Drawing for the job (mm, zero at the part's lowest x, y, z). Coordinates: 2 decimals unless noted, no trailing zeros. Order: outer loops, then holes, each group sorted by start corner. A loop starts at its lowest first (then second) coordinate and runs counter-clockwise, first axis right, second up.
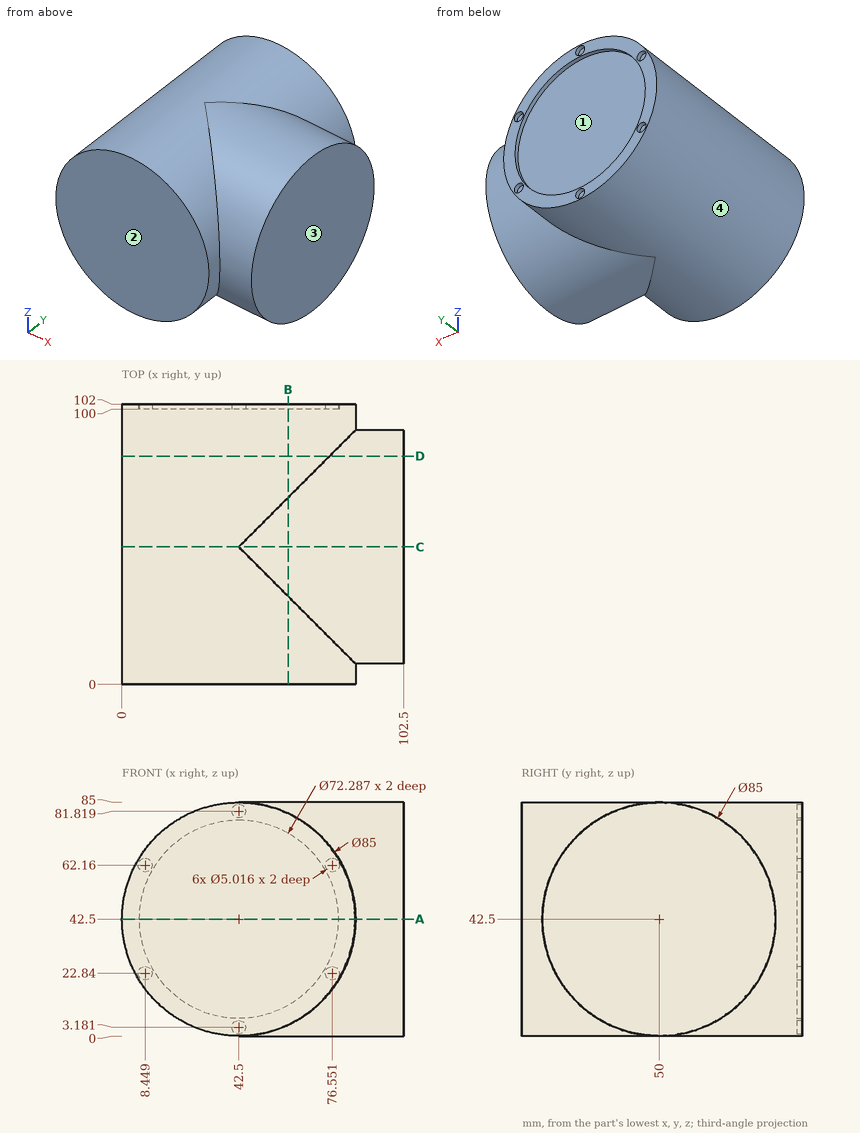
1) Drill centre lines: probe 1 along X at (y, z) = (100.7, 42.5); probe 2 along X at (y, z) = (57.5, 42); probe 3 along Y at (x, z) = (15.5, 40). Where is each one in solid material? Low to high.
2) Slice it at D-D (y = 83). List the corners of the cut face in (x, z).
3) Slice it at B-B (x = 60.5). List the corners of the cut face in (y, z).
4) Slice it at A-A (z = 42.5). List the corners of the cut face in (x, y), plus the area to 3 significant figures.
5) Pin check, flat tips, straight feed: P1, Ø1.5, axis at x = 43, z = 2, coming from the +Y side; P2, Ø1, axis at y = 67, z = 41.5, coming from the -X side; P3, Ø8, axis at x = 85, z = 65.5, coming from the -Y side. Stop position of each tip, or through.
6) Slice it at C-C (y = 50). List the corners of the cut face in (x, z), plus the area to 3 significant figures.
7) Two-plate mould, pull along X, no slides. Class the marked faces 1, 2, 3 and 4: released by +X, released by -X, zero draft, split by the parting line, or undercut.
Worked out:
1. probe 1: x = 0 to 6.36, 78.64 to 85
1. probe 2: x = 0 to 102.5
1. probe 3: y = 0 to 100
2. outline: (75.5, 15.72) - (102.5, 15.72) - (102.5, 69.28) - (75.5, 69.28) arc R42.5 ccw (long way) to start
3. outline: (0, 4) - (32, 4) arc R42.5 ccw to (68, 4) - (102, 4) - (102, 11.16) - (100, 11.16) - (100, 73.84) - (102, 73.84) - (102, 81) - (68, 81) arc R42.5 ccw to (32, 81) - (0, 81) - close
4. outline: (0, 0) - (85, 0) - (85, 7.5) - (102.5, 7.5) - (102.5, 92.5) - (85, 92.5) - (85, 102) - (78.64, 102) - (78.64, 100) - (6.36, 100) - (6.36, 102) - (0, 102) - close
4. area: 10,000 mm2
5. P1: stops at y = 100
5. P2: stops at x = 0
5. P3: stops at y = 11.98
6. outline: (42.5, 0) - (102.5, 0) - (102.5, 85) - (42.5, 85) arc R42.5 ccw to start
6. area: 7,940 mm2
7. face 1: undercut
7. face 2: zero draft
7. face 3: released by +X
7. face 4: split by the parting line
